from build123d import *

# Parameters (mm, degrees)
BOSS_EXTRUDE1_DEPTH = 20
BOSS_EXTRUDE2_DEPTH = 5
FILLET1_R           = 2
SKETCH4_W           = 10
SKETCH4_H           = 10
CUT_EXTRUDE1_DEPTH  = 8.75
SKETCH5_R           = 1.5
CUT_EXTRUDE2_DEPTH  = 22
FILLET2_R           = 1.5


with BuildPart() as part:
    # Sketch1 → Boss-Extrude1 (new body)
    with BuildSketch(Plane.XY):
        Polygon((-130, -28), (-148, -28), (-148, -36.75), (-136, -36.75), (-136, -59.25), (-148, -59.25), (-148, -68), (-130, -68), align=None)
    extrude(amount=-BOSS_EXTRUDE1_DEPTH)

    # Sketch3 → Boss-Extrude2 (add)
    with BuildSketch(Plane(origin=(0, 0, -20), x_dir=(-1, 0, 0), z_dir=(0, 0, -1))):
        with BuildLine():
            Line((155, -73), (130, -73))
            ThreePointArc((130, -73), (127.878679656, -72.121320344), (127, -70))
            Line((127, -70), (127, -26))
            ThreePointArc((127, -26), (127.878679656, -23.878679656), (130, -23))
            Line((130, -23), (155, -23))
            ThreePointArc((155, -23), (157.121320344, -23.878679656), (158, -26))
            Line((158, -26), (158, -70))
            ThreePointArc((158, -70), (157.121320344, -72.121320344), (155, -73))
        make_face()
    extrude(amount=BOSS_EXTRUDE2_DEPTH)

    # Fillet1
    fillet1_edges = [part.edges().sort_by_distance(p)[0] for p in [
        (-130, -68, -10),
        (-130, -28, -10),
    ]]
    fillet(fillet1_edges, radius=FILLET1_R)

    # Sketch4 → Cut-Extrude1 (cut)
    with BuildSketch(Plane.XZ.offset(68)):
        with Locations((-143, -15)):
            Rectangle(SKETCH4_W, SKETCH4_H)
    extrude(amount=-CUT_EXTRUDE1_DEPTH, mode=Mode.SUBTRACT)

    # Sketch5 → Cut-Extrude2 (cut, through all)
    with BuildSketch(Plane.ZY.offset(148)):
        with Locations((-5, -32.375)):
            Circle(SKETCH5_R)
        with Locations((-15, -32.375)):
            Circle(SKETCH5_R)
        with Locations((-5, -63.625)):
            Circle(SKETCH5_R)
    extrude(amount=-CUT_EXTRUDE2_DEPTH, mode=Mode.SUBTRACT)

    # Fillet2
    fillet2_edges = [part.edges().sort_by_distance(p)[0] for p in [
        (-157.121320344, -72.121320344, -20),
        (-158, -48, -20),
        (-157.121320344, -23.878679656, -20),
        (-142.5, -23, -20),
        (-127.878679656, -23.878679656, -20),
        (-127, -48, -20),
        (-127.878679656, -72.121320344, -20),
        (-142.5, -73, -20),
        (-130, -48, 0),
        (-140, -28, 0),
        (-130.585786438, -67.414213562, 0),
        (-130.585786438, -28.585786438, 0),
        (-140, -68, 0),
    ]]
    fillet(fillet2_edges, radius=FILLET2_R)


solid = part.part
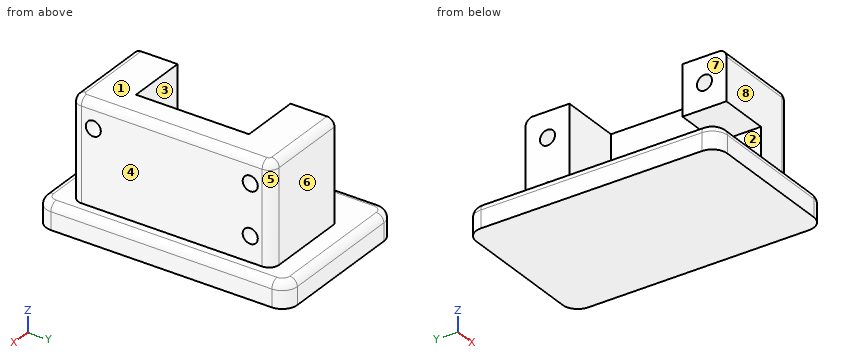
The listing builds one solid part. Answer for the finished solid, in the listing's coordinates (mm). Face numbers are marked on the shaded views. A direction names the side the tool comes from. Coordinates: 2 decimals unless noted, no trailing zeros. Order: outer loops, then holes, each group sorted by start corner. A loop starts at its lowest first (then second) coordinate and runs counter-clockwise, first axis right, second up. Notation, with made-up numbers: (13.5, 34.25) -> (56.5, 34.25) arc R22 ccw to (56.5, 42.25) -> close; hole circle Ø5 at (50, 61). An arc over 180 degrees is marked (long way). Answer in a Markdown table with one row per item. Add a question column.
Item 1: Find section B-B (x = -140). Write down the section's boundary in (y, z) (3 decimals), then the cut area to 3 significant figures.
Item 2: Which of the six approach directions +Z, -Z, +X, -X, +Y, -Y give full straight-line access (tool end or side, diameter ignored) to the marked faces 4, 5, 6, 7 and 8?
Item 3: Find section D-D (y = -53.5). Write down the section's boundary in (x, z).
Item 4: Find section C-C (z = -15). Write down the section's boundary in (x, y) (3 decimals), then the cut area to 3 significant figures.
Item 5: Determine the mould class of the marked faces 1, 2 and 3 for opening direction Z: +Z half, -Z half, draft (parallel to the pull), parting line (faces both ways), or undercut.
Item 6: Find section A-A (z = -5). Write down the section's boundary in (x, y) (3 decimals).
Item 7: Each of these flat-tipped pins is pushed along its axis until it touches: P1, Ø8.5, axis at x = -148.5, y = -53, coming from the +Z side; P2, Ø3, axis at y = -66, z = -7, coming from the -X side; P3, Ø5, axis at y = -43.5, z = -15, coming from the +X side; P4, Ø2, axis at x = -130.5, y = -53, coming from the +Z side. Where does it stop, or does it pass through?
Item 8: Find the intervals of material crossed by L1, parallel to Y at x = -134, z = -5 (3 decimals); L2, parallel to Y at x = -140.75, z = -5 (3 decimals); L3, parallel to Y at x = -140.25, z = -15 (3 decimals), in increasing order. Write a range as from..to.
Result set:
| question | item | result |
|---|---|---|
| 1 | outline | (-73, -25) -> (-23, -25) -> (-23, -21.5) arc R1.5 ccw to (-24.5, -20) -> (-28, -20) -> (-28, -1.5) arc R1.5 ccw to (-29.5, 0) -> (-36.75, 0) -> (-36.75, -20) -> (-71.5, -20) arc R1.5 ccw to (-73, -21.5) -> close; (-68, -10) -> (-59.25, -10) -> (-59.25, 0) -> (-66.5, 0) arc R1.5 ccw to (-68, -1.5) -> close; hole circle Ø3 at (-63.625, -5); hole circle Ø3 at (-32.375, -15); hole circle Ø3 at (-32.375, -5) |
| 1 | area | 489 mm² |
| 2 | face 4 | +Z, +X, +Y, -Y |
| 2 | face 5 | +Z, +X, +Y |
| 2 | face 6 | +Z, +X, -X, +Y |
| 2 | face 7 | +Z, -X, +Y, -Y |
| 2 | face 8 | +Z, +X, -X, -Y |
| 3 | outline | (-158, -25) -> (-127, -25) -> (-127, -21.5) arc R1.5 ccw to (-128.5, -20) -> (-130, -20) -> (-130, -1.5) arc R1.5 ccw to (-131.5, 0) -> (-136, 0) -> (-136, -20) -> (-156.5, -20) arc R1.5 ccw to (-158, -21.5) -> close |
| 4 | outline | (-148, -36.75) -> (-136, -36.75) -> (-136, -59.25) -> (-138, -59.25) -> (-138, -68) -> (-132, -68) arc R2 ccw to (-130, -66) -> (-130, -33.875) -> (-148, -33.875) -> close; (-148, -30.875) -> (-130, -30.875) -> (-130, -30) arc R2 ccw to (-132, -28) -> (-148, -28) -> close |
| 4 | area | 307 mm² |
| 5 | face 1 | +Z half |
| 5 | face 2 | undercut |
| 5 | face 3 | draft |
| 6 | outline | (-148, -68) -> (-132, -68) arc R2 ccw to (-130, -66) -> (-130, -65.125) -> (-148, -65.125) -> close; (-148, -62.125) -> (-130, -62.125) -> (-130, -33.875) -> (-148, -33.875) -> (-148, -36.75) -> (-136, -36.75) -> (-136, -59.25) -> (-148, -59.25) -> close; (-148, -30.875) -> (-130, -30.875) -> (-130, -30) arc R2 ccw to (-132, -28) -> (-148, -28) -> close |
| 7 | P1 | stops at z = -20 |
| 7 | P2 | stops at x = -148 |
| 7 | P3 | stops at x = -130 |
| 7 | P4 | stops at z = 0 |
| 8 | L1 | y = -68..-65.125, -62.125..-33.875, -30.875..-28 |
| 8 | L2 | y = -68..-65.125, -62.125..-59.25, -36.75..-33.875, -30.875..-28 |
| 8 | L3 | y = -36.75..-33.875, -30.875..-28 |
